Check sheet for the modelled part. Datum: model origin and axes. Units: mm. A direction names the side the tool comes from. Give positions to 0.01 mm unless a question says otherwise; leave off trailing zeros. Loops run counter-clockwise (first coordinate to the right, second up) from the corner with the lowest first, then second, coordinate; pieces in that order, holes last. Notation, with made-up numbers: (55, -8.5) - (114, -8.5) arc R18 cw to (114, 4.5) - close; hole circle Ø2 at (-12.5, 89). An arc over 180 degrees is marked (long way). Use CSV: the item, a comma, the result in double quotes.
from build123d import *

# Parameters (mm, degrees)
SKETCH011_R   = 0.825
PAD011_DEPTH  = 65.5
PAD001_DEPTH  = 3
SKETCH002_W   = 16
SKETCH002_H   = 16
PAD002_DEPTH  = 12
SKETCH003_R   = 1.5
PAD003_DEPTH  = 3
SKETCH004_R   = 8
PAD004_DEPTH  = 32
SKETCH005_R   = 12
PAD005_DEPTH  = 1
ARRAY_Z_COUNT = 10
ARRAY_Z_PITCH = 3.45
SKETCH006_R   = 8
PAD006_DEPTH  = 2.3
SKETCH007_R   = 8
PAD007_DEPTH  = 1
SKETCH008_R   = 5.9
PAD008_DEPTH  = 2.3
SKETCH009_R   = 5.9
PAD009_DEPTH  = 5.7
SKETCH010_R   = 5.9
PAD010_DEPTH  = 3.7
SKETCH_R      = 8
PAD_DEPTH     = 3.5


with BuildPart() as pad011:
    # Sketch011 → Pad011 (new body)
    with BuildSketch(Plane.XY.offset(5)):
        Circle(SKETCH011_R)
    extrude(amount=PAD011_DEPTH)


with BuildPart() as cone:
    # Cone → Cone (revolve)
    with BuildSketch(Plane.XZ):
        Polygon((0, 0), (0.2, 0), (2.5, 2), (0, 2), align=None)
    revolve(axis=Axis((0, 0, 0), (0, 0, 1)))


with BuildPart() as pad001:
    # Sketch001 → Pad001 (new body)
    with BuildSketch(Plane.XY.offset(2)):
        Polygon((1.9, -3.290897), (3.8, 0), (1.9, 3.290897), (-1.9, 3.290897), (-3.8, 0), (-1.9, -3.290897), align=None)
    extrude(amount=PAD001_DEPTH)


with BuildPart() as pad002:
    # Sketch002 → Pad002 (new body)
    with BuildSketch(Plane.XY.offset(5)):
        with Locations((0, 3)):
            Rectangle(SKETCH002_W, SKETCH002_H)
    extrude(amount=PAD002_DEPTH)


with BuildPart() as pad003:
    # Sketch003 → Pad003 (new body)
    with BuildSketch(Plane.XY.offset(17)):
        Circle(SKETCH003_R)
    extrude(amount=PAD003_DEPTH)


with BuildPart() as pad004:
    # Sketch004 → Pad004 (new body)
    with BuildSketch(Plane.XY.offset(20)):
        Circle(SKETCH004_R)
    extrude(amount=PAD004_DEPTH)


with BuildPart() as array:
    # Sketch005 → Pad005 (new body)
    with BuildSketch(Plane.XY.offset(20)):
        Circle(SKETCH005_R)
    extrude(amount=PAD005_DEPTH)

    # Array Z: Array ×10


with BuildPart() as array_1:
    add(array.part)
    with Locations(*[(0, 0, i * ARRAY_Z_PITCH) for i in range(1, ARRAY_Z_COUNT)]):
        add(array.part)


with BuildPart() as top03:
    # Sketch006 → Pad006 (new body)
    with BuildSketch(Plane.XY.offset(59)):
        Circle(SKETCH006_R)
    extrude(amount=PAD006_DEPTH)


with BuildPart() as top05:
    # Sketch007 → Pad007 (new body)
    with BuildSketch(Plane.XY.offset(55.7)):
        Circle(SKETCH007_R)
    extrude(amount=PAD007_DEPTH)


with BuildPart() as top04:
    # Sketch008 → Pad008 (new body)
    with BuildSketch(Plane.XY.offset(56.7)):
        Circle(SKETCH008_R)
    extrude(amount=PAD008_DEPTH)


with BuildPart() as top02:
    # Sketch009 → Pad009 (new body)
    with BuildSketch(Plane.XY.offset(61.3)):
        Circle(SKETCH009_R)
    extrude(amount=PAD009_DEPTH)


with BuildPart() as top06:
    # Sketch010 → Pad010 (new body)
    with BuildSketch(Plane.XY.offset(52)):
        Circle(SKETCH010_R)
    extrude(amount=PAD010_DEPTH)


with BuildPart() as cut:
    # Sketch → Pad (new body)
    with BuildSketch(Plane.XY.offset(67)):
        Circle(SKETCH_R)
    extrude(amount=PAD_DEPTH)

    # Fusion: union Cone, Pad001, Pad002, Pad003, Pad004, Array, Top03, Top05, Top04, Top02, Top06
    add(cone.part)
    add(pad001.part)
    add(pad002.part)
    add(pad003.part)
    add(pad004.part)
    add(array_1.part)
    add(top03.part)
    add(top05.part)
    add(top04.part)
    add(top02.part)
    add(top06.part)

    # Cut: cut Pad011
    add(pad011.part, mode=Mode.SUBTRACT)


solid = cut.part
1. Release check for a two-part mould opening along Y. For faces 1 (the face through (-1.73, -7.81, 42.91)), 2 (the face through (-0.608, 0.558, 37.292)), 3 (the face through (-2.863, -1.622, 3.479)) record: released by +Y, released by -Y, zero draft, split by the parting line, or undercut.
Completed:
face 1,"split by the parting line"
face 2,"undercut"
face 3,"released by -Y"
2. Sectioned sample at A-A, the plane z = 11. Record the boundary of the cut face in (x, y) (3 decimals).
Completed:
outline,"(-8, -5) - (8, -5) - (8, 11) - (-8, 11) - close; hole circle Ø1.65 at (0, 0)"
3. Go/stop test with flat-tipped pins: pin 1 Ø5 at (y, z) = (5, 48.5) entering from +X; pin 2 Ø3 at (x, z) = (8.5, 9) entering from -Y; pin 3 Ø5 at (x, z) = (6, 8) entering from +Y. Record where each tip stops, or that it passes through.
Completed:
pin 1,"stops at x = 11.74"
pin 2,"stops at y = -5"
pin 3,"stops at y = 11"
4. Scan lines: line 1 along Z through (x, y) = (-6.75, -2); line 2 along Z through (x, y) = (-3.5, -3); line 3 along Y through (x, z) = (0, 35) (3 decimals). Record each from-to range of solid material in increasing order.
Completed:
line 1,"z = 5 to 17, 20 to 52.05, 55.7 to 56.7, 59 to 61.3, 67 to 70.5"
line 2,"z = 5 to 17, 20 to 70.5"
line 3,"y = -8 to -0.825, 0.825 to 8"
5. Set-up check for faces 4 (the face through (-2.837, 1.668, 3.479)), 5 (the face through (2, -8, 31.35)), 6 (the face through (8, 3, 11)), 7 (the face through (0, -5, 11)), 8 (the face through (3, 0, 2)): record each of +Z, -Z, +X, -X, +Y, -Y from which the full face is reachable in a straight line by a thin tool's end or side.
Completed:
face 4,"-Z, -X, +Y"
face 5,"none"
face 6,"-Z, +X, +Y, -Y"
face 7,"-Z, +X, -X, -Y"
face 8,"-Z"
